```python
from build123d import *

# Parameters (mm, degrees)
ESQUISSE1_R                  = 18.5
BOSS_EXTRU_1_DEPTH           = 24.5
ESQUISSE2_R                  = 15
BOSS_EXTRU_2_DEPTH           = 55
ESQUISSE3_R                  = 6
BOSS_EXTRU_3_DEPTH           = 7
ESQUISSE4_R                  = 3
BOSS_EXTRU_4_DEPTH           = 15.3
ENL_V_START                  = -12
ENL_V_MAT_EXTRU_1_DEPTH      = 12
R_P_TITION_CIRCULAIRE1_COUNT = 6


with BuildPart() as part:
    # Esquisse1 → Boss.-Extru.1 (new body)
    with BuildSketch(Plane(origin=(0, 0, 0), x_dir=(1, 0, 0), z_dir=(0, 1, 0))):
        with Locations(Location((0, 0, 0), (0, 0, 270))):
            Circle(ESQUISSE1_R)
    extrude(amount=BOSS_EXTRU_1_DEPTH)

    # Esquisse2 → Boss.-Extru.2 (add)
    with BuildSketch(Plane(origin=(0, 24.5, 0), x_dir=(1, 0, 0), z_dir=(0, 1, 0))):
        with Locations(Location((0, 0, 0), (0, 0, 270))):
            Circle(ESQUISSE2_R)
    extrude(amount=BOSS_EXTRU_2_DEPTH)

    # Esquisse3 → Boss.-Extru.3 (add)
    with BuildSketch(Plane(origin=(0, 0, 0), x_dir=(1, 0, 0), z_dir=(0, 1, 0))):
        with Locations(Location((0, -7, 0), (0, 0, 270))):
            Circle(ESQUISSE3_R)
    extrude(amount=-BOSS_EXTRU_3_DEPTH)

    # Esquisse4 → Boss.-Extru.4 (add)
    with BuildSketch(Plane.XZ.offset(7)):
        with Locations(Location((0, 7, 0), (0, 0, 270))):
            Circle(ESQUISSE4_R)
    extrude(amount=BOSS_EXTRU_4_DEPTH)

    # Esquisse5 → Enlèv. mat.-Extru.1 (cut)
    with BuildSketch(Plane.XZ.offset(22.3).offset(ENL_V_START)):
        with BuildLine():
            Line((-1.731328969, 4.55), (1.731328969, 4.55))
            ThreePointArc((1.731328969, 4.55), (0, 4), (-1.731328969, 4.55))
        make_face()
    extrude(amount=ENL_V_MAT_EXTRU_1_DEPTH, mode=Mode.SUBTRACT)

    # Esquisse7 → Trou taraudé M31 (revolve, cut)
    with BuildSketch(Plane(origin=(15.5, 0, 0), x_dir=(0, 0, -1), z_dir=(1, 0, 0))):
        Polygon((0, 0), (0, 5.751075774), (1.25, 5), (1.25, 0), align=None)
    trou_taraud_m31 = revolve(axis=Axis((15.5, -6.35, 0), (0, 1, 0)), mode=Mode.SUBTRACT)

    # Répétition circulaire1: Trou taraudé M31 ×6 about axis
    r_p_tition_circulaire1_axis = Axis((0, 0, 0), (0, 1, 0))
    for i in range(1, R_P_TITION_CIRCULAIRE1_COUNT):
        add(trou_taraud_m31.rotate(r_p_tition_circulaire1_axis, i * 360 / R_P_TITION_CIRCULAIRE1_COUNT), mode=Mode.SUBTRACT)


solid = part.part
```
Geometry check sheet. Reference: the model listing, model coordinates, mm. A direction names the side the tool comes from. Round coordinates to 2 decimals unless told otherwise and drop trailing zeros. Loops run counter-clockwise (first coordinate to the right, second up) from the corner with the lowest first, then second, coordinate; pieces in that order, holes last. Notation, with made-up numbers: (72, 59) - (104, 59) arc R27 cw to (104, 75) - close; hole circle Ø8 at (75.5, -24.75). An arc over 180 degrees is marked (long way). Write each question's results on one line, items separated by ' | '. Start each with the question number.
Q1. Access from +Z, -Z, +X, -X, +Y, -Y to the whole of each face (thin tool, end or side, straight path). Record for faces 1 (the cylindrical face through (8.804, 2.465, -12.751)), 2 (the cylindrical face through (-7.086, 12.078, 17.089)), 3 (the cylindrical face through (0.66, 51.615, -14.985)).
Q2. Thickness scan on line 1 (Y direction, x = -13, z = -7); line 2 (Y direction, x = 13, z = -11); line 3 (Z direction, x = 1, y = 23). Record the ranges inside material, lowest first. Write a range as [from, to].
Q3. Release check for a two-part mould opening along Z. For faces 4 (the flat face through (0, -16, 4.55)), 5 (the cylindrical face through (14.26, 2.46, 0.16)), 6 (the flat face through (-1, -7, 4)) record: +Z half, -Z half, draft (parallel to the pull), parting line (faces both ways), or undercut.
Q4. Cross-section at D-D on y = -15. Enter the section's corners in (x, z).
Q5. Gauge pin test, flat ends, axial feed: P1, Ø4, axis at x = 5.5, y = 11.5, coming from the +Z side; P2, Ø12, axis at x = 2.5, y = 58, coming from the -Z side; P3, Ø3, axis at x = -7.75, z = 13.42, coming from the -Y side. Record the tip position at first contact, or that the pin passes through.
Q6. Cross-section at A-A on x = 0. Enter the section's corners in (y, z), and give its area (3 significant figures).
Q7. Cross-section at C-C on z = 8. Enter the section's corners in (x, y).
Q8. Cross-section at B-B on y = 49. Enter the section's corners in (x, z).
Answers below:
1) face 1: -Y | face 2: +Y, -Y | face 3: +Y
2) line 1: y = [0, 79.5] | line 2: y = [0, 24.5] | line 3: z = [-18.47, 18.47]
3) face 4: -Z half | face 5: undercut | face 6: draft
4) outline: (-1.73, 4.55) - (1.73, 4.55) arc R3 ccw (long way) to start
5) P1: stops at z = 18.17 | P2: stops at z = -15 | P3: stops at y = 0
6) outline: (-22.3, 4.55) - (-10.3, 4.55) - (-10.3, 4) - (-7, 4) - (-7, 1) - (0, 1) - (0, -18.5) - (24.5, -18.5) - (24.5, -15) - (79.5, -15) - (79.5, 15) - (24.5, 15) - (24.5, 18.5) - (0, 18.5) - (0, 13) - (-7, 13) - (-7, 10) - (-22.3, 10) - close | area: 2,730 mm²
7) outline: (-16.68, 0) - (-5.92, 0) - (-5.92, -7) - (-2.83, -7) - (-2.83, -22.3) - (2.83, -22.3) - (2.83, -7) - (5.92, -7) - (5.92, 0) - (16.68, 0) - (16.68, 24.5) - (12.69, 24.5) - (12.69, 79.5) - (-12.69, 79.5) - (-12.69, 24.5) - (-16.68, 24.5) - close
8) outline: circle Ø30 at (0, 0)
